from build123d import *

# Parameters (mm, degrees)
SKETCH1_R               = 10
BOSS_EXTRUDE1_DEPTH     = 25
BOSS_EXTRUDE2_DEPTH     = 15
SKETCH4_R               = 4
CUT_EXTRUDE2_DEPTH      = 20
CUT_EXTRUDE2_DEPTH_BACK = 20
SKETCH5_R               = 7.5
CUT_EXTRUDE3_DEPTH      = 20
SKETCH6_R               = 2.5
CUT_EXTRUDE4_DEPTH      = 10
CUT_EXTRUDE4_DEPTH_BACK = 10
SKETCH7_W               = 3
SKETCH7_H               = 18
CUT_EXTRUDE5_DEPTH      = 20


with BuildPart() as part:
    # Sketch1 → Boss-Extrude1 (new body)
    with BuildSketch(Plane(origin=(0, 0, 0), x_dir=(1, 0, 0), z_dir=(0, 1, 0))):
        with Locations(Location((0, 0, 0), (0, 0, 270))):
            Circle(SKETCH1_R)
    extrude(amount=BOSS_EXTRUDE1_DEPTH)

    # Sketch3 → Boss-Extrude2 (add)
    with BuildSketch(Plane(origin=(0, 0, 0), x_dir=(1, 0, 0), z_dir=(0, 1, 0))):
        with BuildLine():
            Line((-4, 9.16515139), (-4, -9.16515139))
            ThreePointArc((-4, -9.16515139), (-10, 0), (-4, 9.16515139))
        make_face()
        with BuildLine():
            Line((4, 9.16515139), (4, -9.16515139))
            ThreePointArc((4, -9.16515139), (10, 0), (4, 9.16515139))
        make_face()
    extrude(amount=-BOSS_EXTRUDE2_DEPTH)

    # Sketch4 → Cut-Extrude2 (cut, two sides)
    with BuildSketch(Plane(origin=(0, 0, 0), x_dir=(0, 0, -1), z_dir=(1, 0, 0))) as cut_extrude2_sk:
        with Locations(Location((0, -7.5, 0), (0, 0, 180))):
            Circle(SKETCH4_R)
        with BuildLine():
            Line((9.25, -7.5), (14.844368797, -7.5))
            Line((14.844368797, -7.5), (14.844368797, -20.157267439))
            Line((14.844368797, -20.157267439), (-15.402777655, -20.157267439))
            Line((-15.402777655, -20.157267439), (-15.402777655, -7.5))
            Line((-15.402777655, -7.5), (-9.25, -7.5))
            ThreePointArc((-9.25, -7.5), (0, -16.75), (9.25, -7.5))
        make_face()
    extrude(amount=CUT_EXTRUDE2_DEPTH, mode=Mode.SUBTRACT)
    extrude(cut_extrude2_sk.sketch, amount=-CUT_EXTRUDE2_DEPTH_BACK, mode=Mode.SUBTRACT)

    # Sketch5 → Cut-Extrude3 (cut)
    with BuildSketch(Plane(origin=(0, 25, 0), x_dir=(1, 0, 0), z_dir=(0, 1, 0))):
        with Locations(Location((0, 0, 0), (0, 0, 270))):
            Circle(SKETCH5_R)
    extrude(amount=-CUT_EXTRUDE3_DEPTH, mode=Mode.SUBTRACT)

    # Sketch6 → Cut-Extrude4 (cut, two sides)
    with BuildSketch(Plane.XY) as cut_extrude4_sk:
        with Locations(Location((0, 19, 0), (0, 0, 180))):
            Circle(SKETCH6_R)
    extrude(amount=CUT_EXTRUDE4_DEPTH, mode=Mode.SUBTRACT)
    extrude(cut_extrude4_sk.sketch, amount=-CUT_EXTRUDE4_DEPTH_BACK, mode=Mode.SUBTRACT)

    # Sketch7 → Cut-Extrude5 (cut)
    with BuildSketch(Plane(origin=(0, 25, 0), x_dir=(1, 0, 0), z_dir=(0, 1, 0))):
        Rectangle(SKETCH7_W, SKETCH7_H)
    extrude(amount=-CUT_EXTRUDE5_DEPTH, mode=Mode.SUBTRACT)


solid = part.part
Read the model definition and answer for the solid it produces. Units are mm, in the model's axes. A direction names the side the tool comes from. Round coordinates to 2 decimals unless told otherwise and drop trailing zeros. Write each loop counter-clockwise with the first axis right and the second up, starting at its lowest first coordinate (ties: lowest second). Pieces come first, ordered by that corner, then holes. Notation, with made-up numbers: (-28, 47) - (-2, 47) arc R14 cw to (-2, 55) - close; hole circle Ø8 at (-8.75, 36). An arc over 180 degrees is marked (long way). One line per question, with ' | ' between items. Start each with the question number.
1. Find the intervals of material crossed by probe 1 along Y at (x, z) = (0, -8); probe 2 along X at (y, z) = (10.5, 1); probe 3 along X at (y, z) = (23, -2.5), in increasing order. Write a range as [from, to].
2. Section A-A (y = -7.5) is taken. Determine the outline of the cut face in (x, z).
3. Section D-D (y = 11) is taken. Determine the outline of the cut face in (x, z), and give its area (3 significant figures).
4. Each of these flat-tipped pins is pushed along its axis until it touches: pin 1 (1 mm diameter, centred on x = -6, y = 9.5, fed in from +Z); pin 2 (0.5 mm diameter, centred on y = 24, z = -8.5, fed in from +X); pin 3 (1.8 mm diameter, centred on y = 22, z = 8, fed in from +X). Where does it stop, or does it pass through?
5. Section B-B (x = 0) is taken. Determine the outline of the cut face in (y, z), and give its area (3 significant figures).
6. For a pull along X with two mould halves and no side action, classify faces 4 (the face through (-4, -7.4, -4.2)), 5 (the face through (0, 11, -9)), 6 (the face through (-7, -15, 0)) as +X half, -X half, draft (parallel to the pull), parting line (faces both ways), or undercut.
7. For faces 1 (the face through (0, 0, 0)), 2 (the face through (6.96, -8.701, 3.815)), 3 (the face through (7.5, 15.1, 0.1)), determine the directions among +Z, -Z, +X, -X, +Y, -Y from which every point of the face is accessible in a straight line to the end or side of a thin tool.
8. Section C-C (z = 0) is taken. Determine the outline of the cut face in (x, y).
Filled in:
1) probe 1: [0, 5] | probe 2: [-9.95, -7.43], [7.43, 9.95] | probe 3: [-9.68, -7.07], [7.07, 9.68]
2) outline: (-9.17, -4) arc R10 ccw to (-4, -9.17) - (-4, -4) - close; (-9.17, 4) - (-4, 4) - (-4, 9.17) arc R10 ccw to start; (4, -9.17) arc R10 ccw to (9.17, -4) - (4, -4) - close; (4, 4) - (9.17, 4) arc R10 ccw to (4, 9.17) - close
3) outline: circle Ø20 at (0, 0); hole (-1.5, -9) - (1.5, -9) - (1.5, -7.35) arc R7.5 ccw to (1.5, 7.35) - (1.5, 9) - (-1.5, 9) - (-1.5, 7.35) arc R7.5 ccw to (-1.5, -7.35) - close | area: 128 mm²
4) pin 1: z = 8.35 | pin 2: x = 5.65 | pin 3: x = 7.04
5) outline: (0, -10) - (16.5, -10) - (16.5, -9) - (5, -9) - (5, 9) - (16.5, 9) - (16.5, 10) - (0, 10) - close; (21.5, -10) - (25, -10) - (25, -9) - (21.5, -9) - close; (21.5, 9) - (25, 9) - (25, 10) - (21.5, 10) - close | area: 130 mm²
6) face 4: undercut | face 5: undercut | face 6: draft
7) face 1: +Z, -Z, -Y | face 2: +X, -X | face 3: +Y
8) outline: (-10, -15) - (-4, -15) - (-4, -11.5) - (-10, -11.5) - close; (-10, -3.5) - (-4, -3.5) - (-4, 0) - (4, 0) - (4, -3.5) - (10, -3.5) - (10, 25) - (7.5, 25) - (7.5, 5) - (-7.5, 5) - (-7.5, 25) - (-10, 25) - close; (4, -15) - (10, -15) - (10, -11.5) - (4, -11.5) - close
